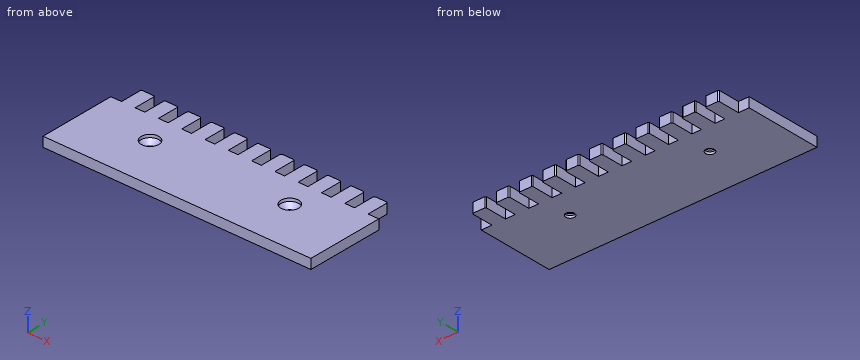
```python
from build123d import *

# Parameters (mm, degrees)
SKETCH_1_W                  = 276
SKETCH_1_H                  = 72
EXTRUDE_1_DEPTH             = 10
CUT_EXTRUDE_1_DEPTH         = 10
SKETCH_6_W                  = 276
SKETCH_6_H                  = 10
EXTRUDE_2_DEPTH             = 30
PATTERN_LINEAR_2_COUNT      = 7
PATTERN_LINEAR_2_PITCH      = 24
PATTERN_LINEAR_2_COUNT_DIR2 = 7
PATTERN_LINEAR_2_PITCH_DIR2 = 24
SKETCH_3_R                  = 4
CUT_EXTRUDE_2_DEPTH         = 10
SKETCH_7_R                  = 9.125
CUT_EXTRUDE_3_DEPTH         = 3
SKETCH_13_W                 = 13.976331663
SKETCH_13_H                 = 30.85518014
SKETCH_13_W_2               = 8.289840829
SKETCH_13_H_2               = 27.158961097
CUT_EXTRUDE_4_DEPTH         = 10


with BuildPart() as part:
    # Эскиз1 → Бобышка-Вытянуть1 (new body)
    with BuildSketch(Plane.XY):
        Rectangle(SKETCH_1_W, SKETCH_1_H)
    extrude(amount=EXTRUDE_1_DEPTH)

    # Эскиз2 → Вырез-Вытянуть1 (cut)
    with BuildSketch(Plane.XY.offset(10)):
        Polygon((-18, 36), (-6, 36), (-7, 35), (-7, 13), (-17, 13), (-17, 35), align=None)
    cut_extrude_1 = extrude(amount=-CUT_EXTRUDE_1_DEPTH, mode=Mode.SUBTRACT)

    # Эскиз6 → Бобышка-Вытянуть2 (add)
    with BuildSketch(Plane.XZ.offset(36)):
        with Locations((0, 5)):
            Rectangle(SKETCH_6_W, SKETCH_6_H)
    extrude(amount=EXTRUDE_2_DEPTH)

    # Линейный массив2: Cut-Extrude 1 7 × 7
    with Locations(*[Vector(1, 0, 0) * (i * PATTERN_LINEAR_2_PITCH) + Vector(-1, 0, 0) * (j * PATTERN_LINEAR_2_PITCH_DIR2) for i in range(PATTERN_LINEAR_2_COUNT) for j in range(PATTERN_LINEAR_2_COUNT_DIR2) if (i, j) != (0, 0)]):
        add(cut_extrude_1, mode=Mode.SUBTRACT)

    # Эскиз3 → Вырез-Вытянуть2 (cut)
    with BuildSketch(Plane.XY.offset(10)):
        with Locations((-72, -16)):
            Circle(SKETCH_3_R)
    cut_extrude_2 = extrude(amount=-CUT_EXTRUDE_2_DEPTH, mode=Mode.SUBTRACT)

    # Эскиз7 → Вырез-Вытянуть3 (cut)
    with BuildSketch(Plane.XY.offset(10)):
        with Locations((-72, -16)):
            Circle(SKETCH_7_R)
    cut_extrude_3 = extrude(amount=-CUT_EXTRUDE_3_DEPTH, mode=Mode.SUBTRACT)

    # Эскиз12 → Зенковка для винта с потайной головкой и внутренним шестигранником M82 (revolve, cut)
    with BuildSketch(Plane(origin=(-72, -16, 7), x_dir=(0, -1, 0), z_dir=(1, 0, 0))):
        Polygon((0, 0), (0, 7), (4.5, 7), (4.5, 4.625), (9.125, 0), align=None)
    hole_wizard_m82 = revolve(axis=Axis((-72, -16, 13.35), (0, 0, -1)), mode=Mode.SUBTRACT)

    # Зеркальное отражение2: Вырез-Вытянуть2, Вырез-Вытянуть3, Зенковка для винта с потайной головкой и внутренним шестигранником M82 across plane
    add(cut_extrude_2.mirror(Plane(origin=(0, 0, 0), x_dir=(0, 0, 1), z_dir=(1, 0, 0))), mode=Mode.SUBTRACT)
    add(cut_extrude_3.mirror(Plane(origin=(0, 0, 0), x_dir=(0, 0, 1), z_dir=(1, 0, 0))), mode=Mode.SUBTRACT)
    add(hole_wizard_m82.mirror(Plane(origin=(0, 0, 0), x_dir=(0, 0, 1), z_dir=(1, 0, 0))), mode=Mode.SUBTRACT)

    # Эскиз13 → Вырез-Вытянуть4 (cut)
    with BuildSketch(Plane.XY.offset(10)):
        with Locations((-143.988165831, 28.42759007)):
            Rectangle(SKETCH_13_W, SKETCH_13_H)
        with Locations((141.144920415, 26.579480549)):
            Rectangle(SKETCH_13_W_2, SKETCH_13_H_2)
    extrude(amount=-CUT_EXTRUDE_4_DEPTH, mode=Mode.SUBTRACT)


solid = part.part
```
Here's how the part is built. I have some questions about the finished solid (model axes, mm). Give positions to 0.01 mm unless a question says otherwise; leave off trailing zeros. Write each loop counter-clockwise with the first axis right and the second up, starting at its lowest first coordinate (ties: lowest second). Pieces come first, ordered by that corner, then holes. Notation, with made-up numbers: (-22, 57) -> (30, 57) arc R35 ccw to (30, 94) -> close; hole circle Ø5 at (44.5, 4.5). An arc over 180 degrees is marked (long way). Write each question's results on one line, items separated by ' | '.
Item 1: Suppose I cut it at A-A on y = -16. Write out the boundary of the cut face in (x, z) (3 decimals).
Output:
outline: (-138, 0) -> (-76.5, 0) -> (-76.5, 2.375) -> (-81.125, 7) -> (-81.125, 10) -> (-138, 10) -> close; (-67.5, 0) -> (67.5, 0) -> (67.5, 2.375) -> (62.875, 7) -> (62.875, 10) -> (-62.875, 10) -> (-62.875, 7) -> (-67.5, 2.375) -> close; (76.5, 0) -> (138, 0) -> (138, 10) -> (81.125, 10) -> (81.125, 7) -> (76.5, 2.375) -> close
Item 2: Suppose I cut it at C-C on x = -10.5. Write out the boundary of the cut face in (y, z).
Output:
outline: (-66, 0) -> (13, 0) -> (13, 10) -> (-66, 10) -> close
Item 3: For pin 1 Ø1.5 at (x, y) = (-64, 22.5) entering from +Z; pin 2 Ø3 at (y, z) = (25, 4.5) entering from -X; pin 3 Ø3 at (y, z) = (25.5, 2.5) entering from +X; pin 4 Ø1.5 at (x, z) = (62, 2) entering from +Y, each with a flat end and sliding along its axis, tell me the tip position at first contact or that it passes through.
Output:
pin 1: passes through | pin 2: stops at x = -127 | pin 3: stops at x = 127 | pin 4: stops at y = 13
Item 4: Suppose I cut it at B-B on x = -72. Write out the boundary of the cut face in (y, z) (3 decimals), plus the area to 3 significant figures.
Output:
outline: (-66, 0) -> (-20.5, 0) -> (-20.5, 2.375) -> (-25.125, 7) -> (-25.125, 10) -> (-66, 10) -> close; (-11.5, 0) -> (36, 0) -> (36, 10) -> (-6.875, 10) -> (-6.875, 7) -> (-11.5, 2.375) -> close | area: 881 mm^2
Item 5: Suppose I cut it at D-D on z = 4.25. Give the number of separate pieces and of enclosed holes in the cut face, plus the area to 3 significant figures.
Output:
separate pieces: 1 | enclosed holes: 2 | area: 25,100 mm^2
Item 6: If I drill on L1, parallel to X at y = -16, z = 8 (3 decimals); L2, parallel to X at y = -16, z = 0.8; L3, parallel to Y at x = 72, z = 7.9 (3 decimals), over which ranges is the centre line in solid material (lowest first)?
Output:
L1: x = -138 to -81.125, -62.875 to 62.875, 81.125 to 138 | L2: x = -138 to -76.5, -67.5 to 67.5, 76.5 to 138 | L3: y = -66 to -25.125, -6.875 to 36
